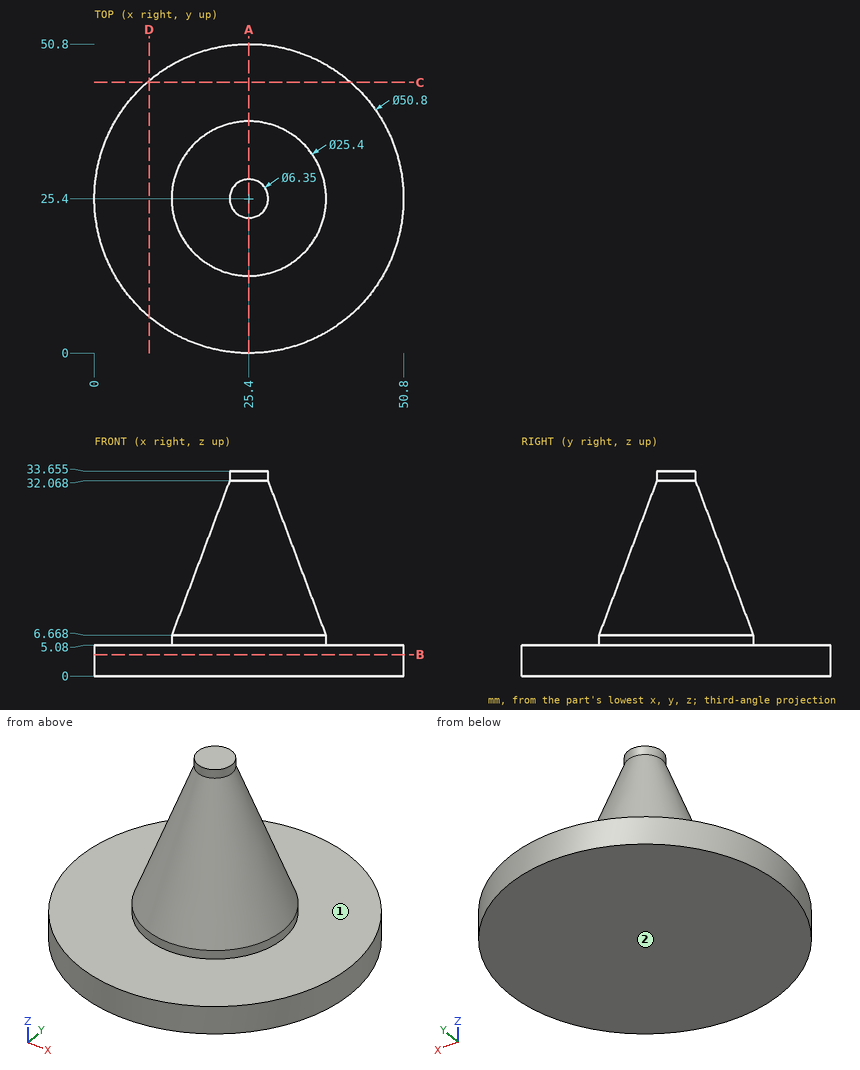
Geometry check sheet. Reference: drawing and pictorial views, mm from the part's lowest x, y, z. A direction names the side the tool comes from. Coordinates: 2 decimals unless noted, no trailing zeros. Order: outer loops, then holes, each group sorted by start corner. A loop starts at its lowest first (then second) coordinate and runs counter-clockwise, first axis right, second up. Notation, with made-up numbers: M 79.25,28 L 129.25,28 A19 ccw 129.25,45 Z; hole C -12.75,61.25 d7. An arc over 180 degrees is marked long. Return JSON: item names as keys, results as strings.
1) Access from +Z, -Z, +X, -X, +Y, -Y to the whole of each face (thin tool, end or side, straight path). Record for the marked faces 1 and 2.
Answer list:
{"face 1": "+Z", "face 2": "-Z, +X, -X, +Y, -Y"}
2) Cross-section at D-D, the plane x = 9. Record the boundary of the cut face in (y, z) (1 decimal), and give its area (3 significant figures).
Answer list:
{"outline": "M 6,0 L 44.8,0 L 44.8,5.1 L 6,5.1 Z", "area": "197 mm2"}
3) Cross-section at C-C, the plane y = 44.5. Record the boundary of the cut face in (x, z).
Answer list:
{"outline": "M 8.66,0 L 42.14,0 L 42.14,5.08 L 8.66,5.08 Z"}
4) Gauge pin test, flat ends, axial feed: pin 1 (3 mm diameter, centred on x = 30.5, z = 15.5, fed in from +Y) (1 decimal); pin 2 (1.5 mm diameter, centred on x = 42, y = 31, fed in from +Z). Record the tip position at first contact, or that the pin passes through.
Answer list:
{"pin 1": "y = 34.3", "pin 2": "z = 5.08"}
5) Thickness scan on L1, parallel to Z at x = 13.5, y = 3.5; L2, parallel to X at y = 16.5, z = 5; L3, parallel to Y at x = 28, z = 21.5. Record the ranges inside material, lowest first. Write a range as [from, to].
Answer list:
{"L1": "[0, 5.08]", "L2": "[1.61, 49.19]", "L3": "[18.75, 32.05]"}
6) Cross-section at B-B, the plane z = 3.5. Record the boundary of the cut face in (x, y).
Answer list:
{"outline": "C 25.4,25.4 d50.8"}
7) Cross-section at A-A, the plane x = 25.4. Record the boundary of the cut face in (y, z) (1 decimal).
Answer list:
{"outline": "M 0,0 L 50.8,0 L 50.8,5.1 L 38.1,5.1 L 38.1,6.7 L 28.6,32.1 L 28.6,33.7 L 22.2,33.7 L 22.2,32.1 L 12.7,6.7 L 12.7,5.1 L 0,5.1 Z"}
